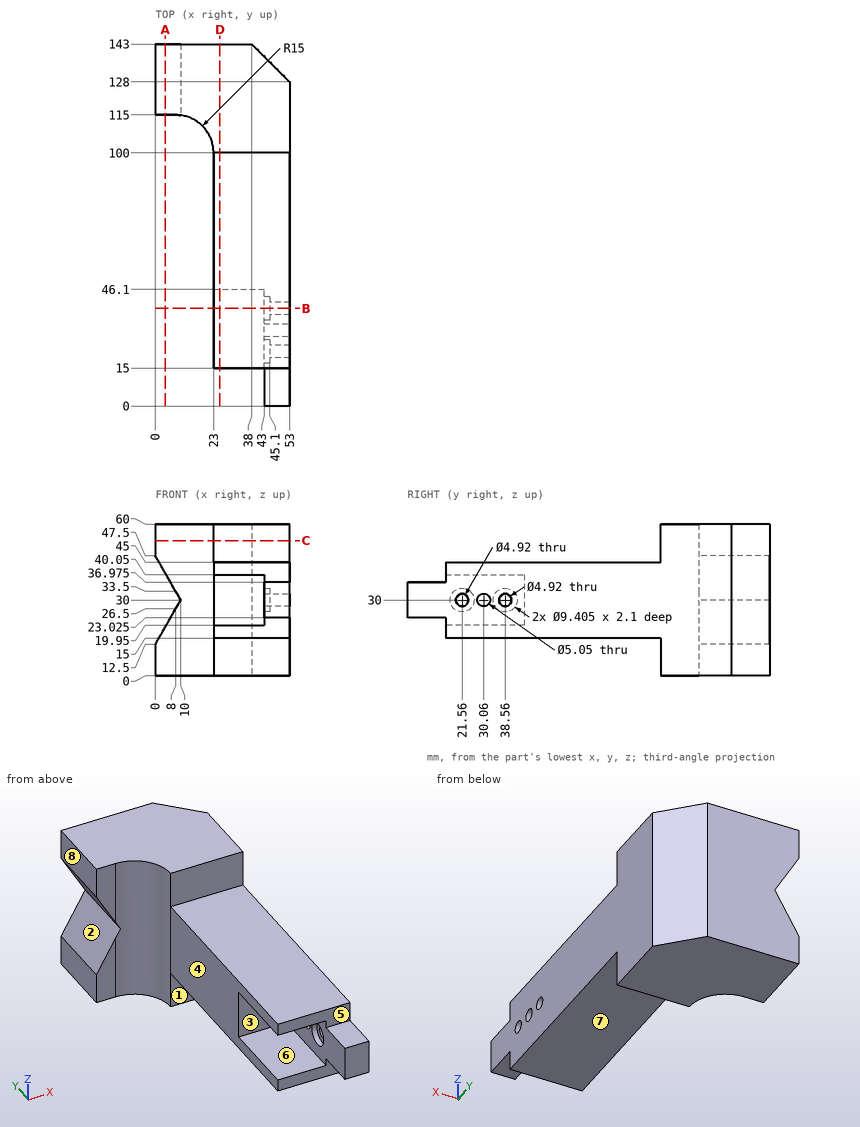
Could you check a few things on this drawing? It's one solid part, dimensions in mm from its lowest x, y, z. A direction names the side the tool comes from. Give positions to 0.01 mm unless a question says otherwise; leave off trailing zeros. Order: outer loops, then holes, each group sorted by start corner. A loop starts at its lowest first (then second) coordinate and runs counter-clockwise, first axis right, second up. Notation, with made-up numbers: (36, 77) -> (54, 77) arc R4 ccw to (54, 84) -> close; hole circle Ø11 at (45, 59.5). An arc over 180 degrees is marked (long way). Use CSV: the item, a comma, the result in double quotes. Start each with the question number.
Item 1: Thinking about a two-plate mould opening in Z: for the marked faces 6, 7 and 8, which applies, pulls with the +Z half, pulls with the -Z half, needs draft (parallel to the pull), parting line crosses it, or undercut?
Item 2: Suppose I cut it at D-D (x = 25.5). List the corners of the cut face in (y, z) for me.
Item 3: On a 3-axis mill with a long thin cutter (end or side, diameter ignored), from which of +Z, -Z, +X, -X, +Y, -Y can I reach the whole of each face in a straight line? I mean the marked faces 1, 2, 3, 4 and 5. Say none if no direction works.
Item 4: I'm going to push flat-ended pins straight in: P1, Ø2.5, axis at x = 3, z = 18.5, coming from the -Y side; P2, Ø12, axis at y = 20, z = 12.5, coming from the +X side; P3, Ø2, axis at y = 117, z = 34.5, coming from the -X side; P4, Ø12, axis at y = 38.56, z = 30, coming from the -X side. Where does each tip first touch, or does it pass through?
Item 5: Suppose I cut it at B-B (y = 38.56). List the corners of the cut face in (x, z) for me, and give its area (3 significant figures).
Item 6: Suppose I cut it at C-C (z = 53.5). List the corners of the cut face in (x, y) for me, and give its area (3 significant figures).
Item 7: If I drill on probe 1 along Z at (x, y) = (50.25, 38.56); probe 2 along Y at (x, z) = (44, 30) (1 decimal); probe 3 along Y at (x, z) = (51, 30) (3 decimals), over which ranges is the centre line in solid material (lowest first)? Write a range as [from, to].
Item 8: Suppose I cut it at A-A (x = 4). List the corners of the cut face in (y, z) for me.
Answer block:
1,face 6,"undercut"
1,face 7,"pulls with the -Z half"
1,face 8,"needs draft"
2,outline,"(15, 15) -> (100, 15) -> (100, 0) -> (143, 0) -> (143, 60) -> (100, 60) -> (100, 45) -> (15, 45) -> (15, 40.05) -> (46.1, 40.05) -> (46.1, 19.95) -> (15, 19.95) -> close"
3,face 1,"-Z, +X, -X, -Y"
3,face 2,"-X, +Y, -Y"
3,face 3,"-X, -Y"
3,face 4,"+Z, -Z, -X, -Y"
3,face 5,"+Z, +X, -X, -Y"
4,P1,"stops at y = 115"
4,P2,"stops at x = 53"
4,P3,"stops at x = 6.86"
4,P4,"stops at x = 43"
5,outline,"(23, 15) -> (53, 15) -> (53, 27.54) -> (45.1, 27.54) -> (45.1, 25.3) -> (43, 25.3) -> (43, 19.95) -> (23, 19.95) -> close; (23, 40.05) -> (43, 40.05) -> (43, 34.7) -> (45.1, 34.7) -> (45.1, 32.46) -> (53, 32.46) -> (53, 45) -> (23, 45) -> close"
5,area,"439 mm^2"
6,outline,"(0, 115) -> (8, 115) arc R15 cw to (23, 100) -> (53, 100) -> (53, 128) -> (38, 143) -> (0, 143) -> close"
6,area,"1,870 mm^2"
7,probe 1,"z = [15, 27.54], [32.46, 45]"
7,probe 2,"y = [0, 16.9], [26.3, 27.5], [32.6, 33.9], [43.3, 137]"
7,probe 3,"y = [0, 19.1], [24.02, 27.535], [32.585, 36.1], [41.02, 130]"
8,outline,"(115, 0) -> (143, 0) -> (143, 19.5) -> (115, 19.5) -> close; (115, 40.5) -> (143, 40.5) -> (143, 60) -> (115, 60) -> close"
